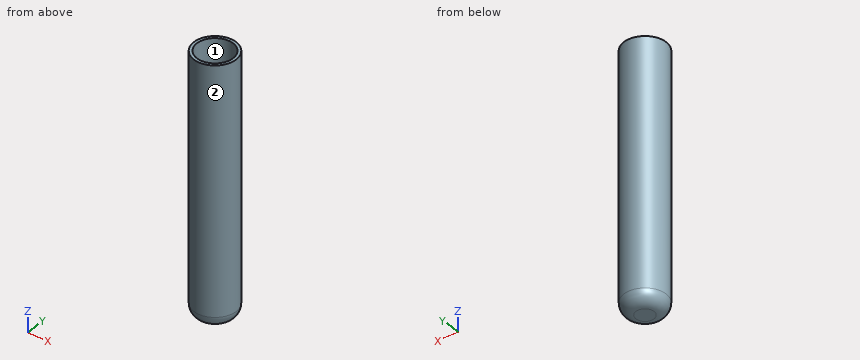
```python
from build123d import *

# Parameters (mm, degrees)
SKETCH_R     = 7
PAD_DEPTH    = 85
SKETCH001_R  = 6
POCKET_DEPTH = 83
FILLET_R     = 4


with BuildPart() as part:
    # Sketch → Pad (new body)
    with BuildSketch(Plane.XY):
        Circle(SKETCH_R)
    extrude(amount=PAD_DEPTH)

    # Sketch001 (on Face3 of Pad) → Pocket (cut)
    with BuildSketch(Plane.XY.offset(85)):
        Circle(SKETCH001_R)
    extrude(amount=-POCKET_DEPTH, mode=Mode.SUBTRACT)

    # Fillet
    fillet_edges = [part.edges().sort_by_distance(p)[0] for p in [
        (-7, 0, 0),
    ]]
    fillet(fillet_edges, radius=FILLET_R)


solid = part.part
```
CAD build for the part. Positions are in the model's coordinates, mm. Face numbers are marked on the shaded views. Coordinates: 2 decimals unless noted, no trailing zeros. Order: outer loops, then holes, each group sorted by start corner. A loop starts at its lowest first (then second) coordinate and runs counter-clockwise, first axis right, second up.
(1) Mould opens along Y. For the marked faces 1 and 2 say: released by +Y, released by -Y, zero draft, split by the parting line, or undercut.
Solution:
face 1: undercut
face 2: split by the parting line
(2) Saw through at A-A, the plane z = 21.5. Write the cut outline in (x, y), and give its area (3 significant figures).
Solution:
outline: circle Ø14 at (0, 0); hole circle Ø12 at (0, 0)
area: 40.8 mm2
(3) Drill centre lines: L1, parallel to Z at x = 0, y = -2; L2, parallel to Y at x = 0, z = 26.5; L3, parallel to Y at x = 4.75, z = 49.5. Where is each one in solid material? Low to high.
Solution:
L1: z = 0 to 2
L2: y = -7 to -6, 6 to 7
L3: y = -5.14 to -3.67, 3.67 to 5.14
(4) Pin check, flat tips, straight feed: pin 1 Ø1.5 at (x, z) = (1.5, 57) entering from -Y; pin 2 Ø1.5 at (x, y) = (-3, -3) entering from -Z; pin 3 Ø1 at (x, y) = (-5, -3) entering from -Z. Stop position of each tip, or through.
Solution:
pin 1: stops at y = -6.96
pin 2: stops at z = 0.03
pin 3: stops at z = 0.75
